```python
from build123d import *

# Parameters (mm, degrees)
SKETCH1_W           = 584.2
SKETCH1_H           = 635
BOSS_EXTRUDE1_DEPTH = 25.4
SKETCH2_W           = 76.2
SKETCH2_H           = 20.32
BOSS_EXTRUDE2_DEPTH = 25.4
SKETCH3_W           = 76.2
SKETCH3_H           = 20.32
BOSS_EXTRUDE3_DEPTH = 25.4
FILLET1_R           = 5.08
FILLET2_R           = 5.08
FILLET3_R           = 5.08
FILLET4_R           = 5.08


with BuildPart() as part:
    # Sketch1 → Boss-Extrude1 (new body)
    with BuildSketch(Plane(origin=(0, 0, 0), x_dir=(1, 0, 0), z_dir=(0, 1, 0))):
        with Locations((292.1, 317.5)):
            Rectangle(SKETCH1_W, SKETCH1_H)
    extrude(amount=BOSS_EXTRUDE1_DEPTH)

    # Sketch2 → Boss-Extrude2 (add)
    with BuildSketch(Plane.XY):
        with Locations((292.1, 15.24)):
            Rectangle(SKETCH2_W, SKETCH2_H)
    extrude(amount=BOSS_EXTRUDE2_DEPTH)

    # Sketch3 → Boss-Extrude3 (add)
    with BuildSketch(Plane(origin=(0, 0, -635), x_dir=(-1, 0, 0), z_dir=(0, 0, -1))):
        with Locations((-292.1, 15.24)):
            Rectangle(SKETCH3_W, SKETCH3_H)
    extrude(amount=BOSS_EXTRUDE3_DEPTH)

    # Fillet1
    fillet1_edges = [part.edges().sort_by_distance(p)[0] for p in [
        (292.1, 25.4, -660.4),
    ]]
    fillet(fillet1_edges, radius=FILLET1_R)

    # Fillet2
    fillet2_edges = [part.edges().sort_by_distance(p)[0] for p in [
        (292.1, 5.08, -660.4),
    ]]
    fillet(fillet2_edges, radius=FILLET2_R)

    # Fillet3
    fillet3_edges = [part.edges().sort_by_distance(p)[0] for p in [
        (292.1, 5.08, 25.4),
    ]]
    fillet(fillet3_edges, radius=FILLET3_R)

    # Fillet4
    fillet4_edges = [part.edges().sort_by_distance(p)[0] for p in [
        (292.1, 25.4, 25.4),
    ]]
    fillet(fillet4_edges, radius=FILLET4_R)


solid = part.part
```
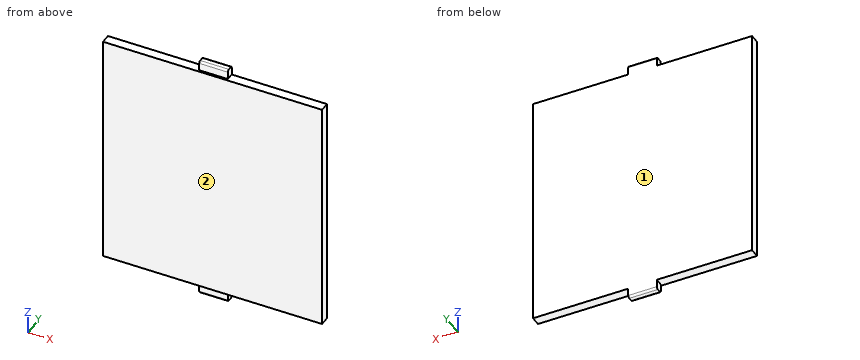
The model under review builds one solid part; all positions refer to its coordinate system, in mm. Face numbers are marked on the shaded views. Round coordinates to 2 decimals unless told otherwise and drop trailing zeros. Loops run counter-clockwise (first coordinate to the right, second up) from the corner with the lowest first, then second, coordinate; pieces in that order, holes last. Notation, with made-up numbers: (-1, 28.5) - (38, 28.5) arc R18 ccw to (38, 52.5) - close; hole circle Ø5 at (-25.5, 70). An arc over 180 degrees is marked (long way). Write each question's results on one line, items separated by ' | '. Start each with the question number.
Q1. Draft analysis for pull direction Y (two halves, no side actions). For the marked faces 1 and 2, state which applies: pulls with the +Y half, pulls with the -Y half, needs draft (parallel to the pull), parting line crosses it, or undercut.
Q2. Take a section at A-A on y = 14.5. Give the boundary of the cut face in (x, z).
Q3. Take a section at C-C on x = 81. Give the boundary of the cut face in (y, z), plus the area to 3 significant figures.
Q4. Insertion check: P1, Ø7.5, axis at x = 365, y = 12.5, coming from the +Z side; P2, Ø6, axis at y = 19, z = -642.5, coming from the +X side; P3, Ø10, axis at y = 12.5, z = -654, coming from the -X side. Each pin has a flat end and moves straight along its axis. Give the tip position at first contact, or say it passes through.
Q5. Wall thickness on line 1 along Z through (x, y) = (353.5, 3.75); line 2 along Z through (x, y) = (316.5, 6): over which ranges is each line inside the solid? List them lowest first. Write a range as [from, to].
Q6. Take a section at B-B on x = 302. Give the boundary of the cut face in (y, z).
Data:
1) face 1: pulls with the +Y half | face 2: pulls with the -Y half
2) outline: (0, -635) - (254, -635) - (254, -660.4) - (330.2, -660.4) - (330.2, -635) - (584.2, -635) - (584.2, 0) - (330.2, 0) - (330.2, 25.4) - (254, 25.4) - (254, 0) - (0, 0) - close
3) outline: (0, -635) - (25.4, -635) - (25.4, 0) - (0, 0) - close | area: 16,100 mm²
4) P1: stops at z = 0 | P2: stops at x = 330.2 | P3: stops at x = 254
5) line 1: z = [-635, 0] | line 2: z = [-658.24, 23.24]
6) outline: (0, -635) - (5.08, -635) - (5.08, -655.32) arc R5.08 ccw to (10.16, -660.4) - (20.32, -660.4) arc R5.08 ccw to (25.4, -655.32) - (25.4, 20.32) arc R5.08 ccw to (20.32, 25.4) - (10.16, 25.4) arc R5.08 ccw to (5.08, 20.32) - (5.08, 0) - (0, 0) - close
